from build123d import *

# Parameters (mm, degrees)
SKETCH_1_W          = 28.9
SKETCH_1_H          = 186
EXTRUDE_1_DEPTH     = 3
FILLET_1_R          = 3
SKETCH_2_R          = 1.5
SKETCH_2_W          = 21.9
SKETCH_2_H          = 12
CUT_EXTRUDE_1_DEPTH = 3
FILLET_2_R          = 3
SKETCH_3_W          = 10
SKETCH_3_H          = 30
CUT_EXTRUDE_2_DEPTH = 3
FILLET_3_R          = 3


with BuildPart() as part:
    # Sketch 1 → Extrude 1 (new body)
    with BuildSketch(Plane(origin=(0, 0, 0), x_dir=(1, 0, 0), z_dir=(0, 1, 0))):
        Rectangle(SKETCH_1_W, SKETCH_1_H)
    extrude(amount=EXTRUDE_1_DEPTH)

    # Fillet 1
    fillet_1_edges = [part.edges().sort_by_distance(p)[0] for p in [
        (14.45, 1.5, 93),
        (-14.45, 1.5, 93),
        (-14.45, 1.5, -93),
        (14.45, 1.5, -93),
    ]]
    fillet(fillet_1_edges, radius=FILLET_1_R)

    # Sketch 2 → Cut-Extrude 1 (cut)
    with BuildSketch(Plane(origin=(0, 3, 0), x_dir=(1, 0, 0), z_dir=(0, 1, 0))):
        with Locations(Location((10, -89.5, 0), (0, 0, 270))):
            Circle(SKETCH_2_R)
        with Locations(Location((-10, -89.5, 0), (0, 0, 90))):
            Circle(SKETCH_2_R)
        with Locations(Location((-10, 89.5, 0), (0, 0, 270))):
            Circle(SKETCH_2_R)
        with Locations(Location((10, 89.5, 0), (0, 0, 90))):
            Circle(SKETCH_2_R)
        with Locations(Location((-5, -38, 0), (0, 0, 270))):
            Circle(SKETCH_2_R)
        with Locations(Location((-5, -62, 0), (0, 0, 270))):
            Circle(SKETCH_2_R)
        with Locations(Location((5, -38, 0), (0, 0, 90))):
            Circle(SKETCH_2_R)
        with Locations(Location((5, -62, 0), (0, 0, 90))):
            Circle(SKETCH_2_R)
        with Locations(Location((5, 62, 0), (0, 0, 270))):
            Circle(SKETCH_2_R)
        with Locations(Location((-5, 62, 0), (0, 0, 90))):
            Circle(SKETCH_2_R)
        with Locations(Location((5, 38, 0), (0, 0, 270))):
            Circle(SKETCH_2_R)
        with Locations(Location((-5, 38, 0), (0, 0, 90))):
            Circle(SKETCH_2_R)
        with Locations(Location((-7.45, 7, 0), (0, 0, 270))):
            Circle(SKETCH_2_R)
        with Locations(Location((-7.45, -7, 0), (0, 0, 90))):
            Circle(SKETCH_2_R)
        with Locations(Location((-5, -68.5, 0), (0, 0, 270))):
            Circle(SKETCH_2_R)
        with Locations(Location((-5, -83.5, 0), (0, 0, 270))):
            Circle(SKETCH_2_R)
        with Locations(Location((5, -83.5, 0), (0, 0, 90))):
            Circle(SKETCH_2_R)
        with Locations(Location((5, -68.5, 0), (0, 0, 90))):
            Circle(SKETCH_2_R)
        with Locations(Location((5, 83.5, 0), (0, 0, 270))):
            Circle(SKETCH_2_R)
        with Locations(Location((-5, 83.5, 0), (0, 0, 90))):
            Circle(SKETCH_2_R)
        with Locations(Location((5, 68.5, 0), (0, 0, 270))):
            Circle(SKETCH_2_R)
        with Locations(Location((-5, 68.5, 0), (0, 0, 90))):
            Circle(SKETCH_2_R)
        with Locations(Location((10.95, 25, 0), (0, 0, 270))):
            Circle(SKETCH_2_R)
        with Locations(Location((10.95, -25, 0), (0, 0, 90))):
            Circle(SKETCH_2_R)
        with Locations(Location((-10.95, -25, 0), (0, 0, 270))):
            Circle(SKETCH_2_R)
        with Locations(Location((-10.95, 25, 0), (0, 0, 90))):
            Circle(SKETCH_2_R)
        with Locations((-3.5, 50)):
            Rectangle(SKETCH_2_W, SKETCH_2_H)
        with Locations((-3.5, -50)):
            Rectangle(SKETCH_2_W, SKETCH_2_H)
    extrude(amount=-CUT_EXTRUDE_1_DEPTH, mode=Mode.SUBTRACT)

    # Fillet 2
    fillet_2_edges = [part.edges().sort_by_distance(p)[0] for p in [
        (-14.45, 1.5, -44),
        (-14.45, 1.5, -56),
        (7.45, 1.5, -56),
        (7.45, 1.5, -44),
        (-14.45, 1.5, 56),
        (-14.45, 1.5, 44),
        (7.45, 1.5, 44),
        (7.45, 1.5, 56),
    ]]
    fillet(fillet_2_edges, radius=FILLET_2_R)

    # Sketch 3 → Cut-Extrude 2 (cut)
    with BuildSketch(Plane(origin=(0, 3, 0), x_dir=(1, 0, 0), z_dir=(0, 1, 0))):
        with Locations((4.45, 0)):
            Rectangle(SKETCH_3_W, SKETCH_3_H)
    extrude(amount=-CUT_EXTRUDE_2_DEPTH, mode=Mode.SUBTRACT)

    # Fillet 3
    fillet_3_edges = [part.edges().sort_by_distance(p)[0] for p in [
        (9.45, 1.5, -15),
        (9.45, 1.5, 15),
        (-0.55, 1.5, 15),
        (-0.55, 1.5, -15),
    ]]
    fillet(fillet_3_edges, radius=FILLET_3_R)


solid = part.part
Can you work these out from the model? Positions are in its coordinate system, mm. A direction names the side the tool comes from. Give positions to 0.01 mm unless a question says otherwise; leave off trailing zeros. Answer as a JSON object with one key per item and string values.
Q1. If I drill on L1, parallel to X at y = 2, z = 89.5; L2, parallel to X at y = 1.05, z = -62; L3, parallel to Z at x = -1.75, y = 2.1, over which ranges is the centre line in solid material (lowest first)?
Geometry says:
{"L1": "-14.45 to -11.5, -8.5 to 8.5, 11.5 to 14.45", "L2": "-14.45 to -6.5, -3.5 to 3.5, 6.5 to 14.45", "L3": "-93 to -56, -44 to 44, 56 to 93"}
Q2. Will this pin go through, and if not, where does the flat tip stop? P1, Ø0.9, axis at y = 1, z = 49, coming from the -X side.
Geometry says:
{"P1": "x = 7.45"}
Q3. Which directions (+Z, -Z, +X, -X, +Y, -Y) give clear straight access to the entire face, cutting with the end or side of a thin tool? Please do faces 1 (the flat face through (-4, 2, -44)), 2 (the flat face through (-3, 3, -1)), 3 (the cylindrical face through (8.55, 1.48, 14.14)).
Geometry says:
{"face 1": "-X, +Y, -Y", "face 2": "+Z, -Z, +X, -X, +Y", "face 3": "+Y, -Y"}
Q4. Imagine slicing it at A-A on y = 1.65. Give the number of separate pieces and of enclosed holes in the cut face, plus the area to 3 significant figures.
Geometry says:
{"separate pieces": "1", "enclosed holes": "27", "area": "4,370 mm²"}
Q5. If we mould it in two halves opening along X, with no side actions, what happens to faces 4 (the flat face through (9.45, 2, 0)), 5 (the cylindrical face through (-13.55, 1.48, -56.86)), 6 (the flat face through (-4, 2, -56))? For each: pulls with the +X half, pulls with the -X half, needs draft (parallel to the pull), parting line crosses it, or undercut.
Geometry says:
{"face 4": "undercut", "face 5": "pulls with the -X half", "face 6": "needs draft"}
